Check sheet for the drawn part. Datum: minimum x, y, z corner. Units: mm. A direction names the side the tool comes from. Coordinates: 2 decimals unless noted, no trailing zeros. Order: outer loops, then holes, each group sorted by start corner. A loop starts at its lowest first (then second) coordinate and runs counter-clockwise, first axis right, second up.
Q1. Set-up check for the marked faces 1 and 2: record each of +Z, -Z, +X, -X, +Y, -Y from which the full face is reachable in a straight line by a thin tool's end or side.
Q2. Cross-section at C-C, the plane y = 46.75. Record the boundary of the cut face in (x, z).
Q3. Draft check along Y on the marked faces 3, 4 and 5. Enter one of: pulls with the +Y half, pulls with the -Y half, needs draft (parallel to the pull), parting line crosses it, or undercut.
Q4. Depth check by flat-ended pin: P1, Ø4.5, axis at y = 12.5, z = 8.5, coming from the +X side; P2, Ø3, axis at y = 31, z = 8, coming from the -X side; P3, Ø1.5, axis at x = 33, z = 13, coming from the -Y side; P4, Ø2, axis at x = 37, y = 29.5, coming from the -Z side. Enter the tip coordinate at first touch or a pass-through.
Q5. Cross-section at D-D, the plane x = 40. Record the boundary of the cut face in (y, z), and give its area (3 significant figures).
Q6. Cross-section at B-B, the plane x = 29. Record the boundary of the cut face in (y, z).
Q7. Cross-section at A-A, the plane z = 5.25. Count the separate pieces of the cut face and the enclosed holes in it, and give its area (3 significant figures).
Q8. Thickness scan on line 1 (Y direction, x = 29, z = 12); line 2 (X direction, y = 40.5, z = 1); line 3 (Y direction, x = 47.5, z = 12.25) (1 decimal). Record the ranges inside material, lowest first.
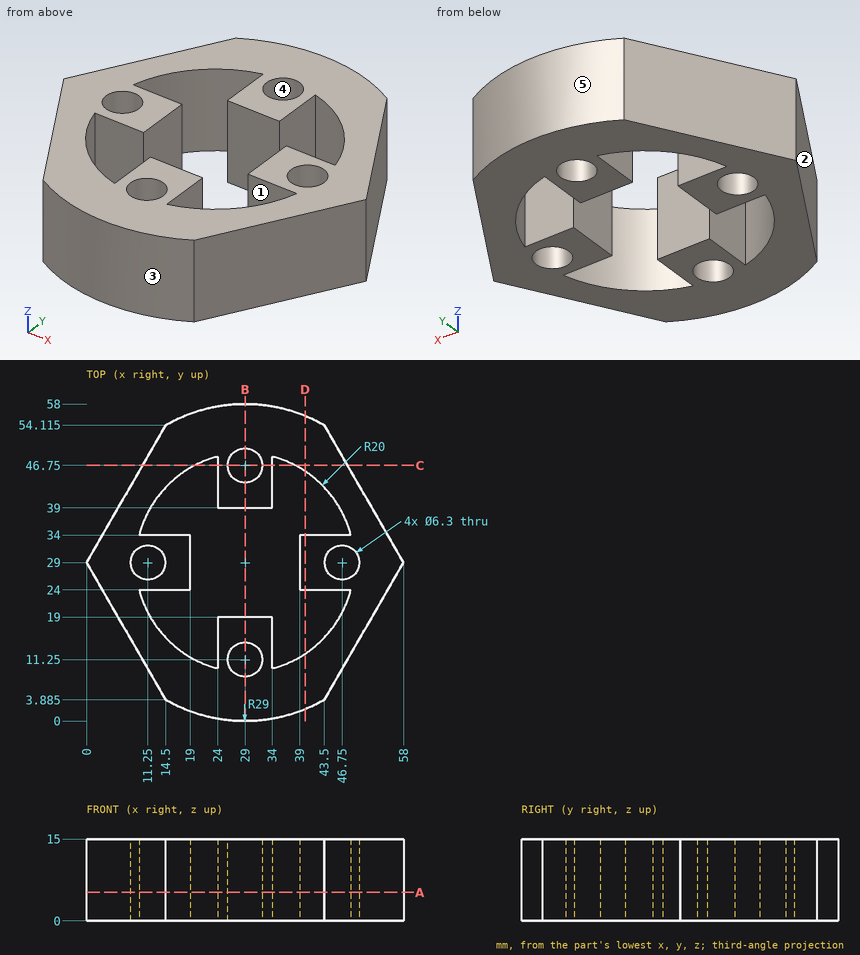
Check values:
1. face 1: +Z, -Z
1. face 2: +Z, -Z, -X, -Y
2. outline: (10.25, 0) - (19.78, 0) - (19.78, 15) - (10.25, 15) - close; (24, 0) - (25.85, 0) - (25.85, 15) - (24, 15) - close; (32.15, 0) - (34, 0) - (34, 15) - (32.15, 15) - close; (38.22, 0) - (47.75, 0) - (47.75, 15) - (38.22, 15) - close
3. face 3: pulls with the -Y half
3. face 4: undercut
3. face 5: pulls with the +Y half
4. P1: stops at x = 49.77
4. P2: stops at x = 0.29
4. P3: stops at y = 0.18
4. P4: passes through
5. outline: (2.17, 0) - (12.3, 0) - (12.3, 15) - (2.17, 15) - close; (24, 0) - (34, 0) - (34, 15) - (24, 15) - close; (45.7, 0) - (55.83, 0) - (55.83, 15) - (45.7, 15) - close
5. area: 454 mm2
6. outline: (0, 0) - (8.1, 0) - (8.1, 15) - (0, 15) - close; (14.4, 0) - (19, 0) - (19, 15) - (14.4, 15) - close; (39, 0) - (43.6, 0) - (43.6, 15) - (39, 15) - close; (49.9, 0) - (58, 0) - (58, 15) - (49.9, 15) - close
7. separate pieces: 1
7. enclosed holes: 5
7. area: 1,350 mm2
8. line 1: y = 0 to 8.1, 14.4 to 19, 39 to 43.6, 49.9 to 58
8. line 2: x = 6.64 to 12.64, 24 to 34, 45.36 to 51.36
8. line 3: y = 10.8 to 21.4, 24 to 25.9, 32.1 to 34, 36.6 to 47.2
